from build123d import *

# Parameters (mm, degrees)
F0_R     = 38.1
F1_DEPTH = 6.35
F2_W     = 23.521014
F2_H     = 14.845229
F3_DEPTH = 5.842
F4_R     = 5.483658
F5_DEPTH = 27.94


with BuildPart() as f1:
    # F0 (on Top) → F1 (new body)
    with BuildSketch(Plane.XY):
        Circle(F0_R)
    extrude(amount=F1_DEPTH)

    # F2 (on face) → F3 (join)
    with BuildSketch(Plane.XY.offset(6.35)):
        with Locations((0.192795, 17.737156)):
            Rectangle(F2_W, F2_H)
    extrude(amount=F3_DEPTH)

    # F4 (on face) → F5 (cut)
    with BuildSketch(Plane.XY.offset(12.192)):
        with Locations((0, 17.833555)):
            Circle(F4_R)
    extrude(amount=-F5_DEPTH, mode=Mode.SUBTRACT)


solid = f1.part
Geometry: final body of the model. Coordinates: model frame, mm. A direction names the side the tool comes from. Round coordinates to 2 decimals unless told otherwise and drop trailing zeros. Loops run counter-clockwise (first coordinate to the right, second up) from the corner with the lowest first, then second, coordinate; pieces in that order, holes last. Notation, with made-up numbers: (41, 69.5) - (96, 69.5) arc R20 ccw to (96, 101.5) - close; hole circle Ø11 at (49.5, 6.25). An arc over 180 degrees is marked (long way). Write each question's results on one line, items separated by ' | '. Start each with the question number.
1) Access query for faces 1 (the face through (11.953, 18, 9)), 2 (the face through (-11.568, 18, 9)), 3 (the face through (0, 10.315, 9)), 4 (the face through (0, 25.16, 9)). Directions: +Z, -Z, +X, -X, +Y, -Y. A direction counts if a zero-diameter tool reaches every point of the face in a straight line with its end or side. Return the directions, or none.
2) Cut plane D-D on x = -10. Return loops of the section in (y, z).
3) Cut plane A-A on x = 0. Return loops of the section in (y, z).
4) Cut plane B-B on y = 0. Return loops of the section in (x, z), then the cut area to 3 significant figures.
5) Cut plane C-C on z = 1.75. Return loops of the section in (x, y), then the cut area to 3 significant figures.
6) Line query: probe 1 along Y at (x, z) = (0, 7.75); probe 2 along Z at (x, y) = (25, 17); probe 3 along Y at (x, z) = (0, 4). Output: solid intervals per line, ascending. Write a range as [from, to].
7) Mould query, pull axis X, two halves, no side actions, for faces 5 (the face through (-1.19, 12.48, 6.18)), 6 (the face through (-30.235, -23.183, 3.131)), 7 (the face through (-1, 1, 6.35)). Classes: released by +X, released by -X, zero draft, split by the parting line, or undercut.
8) First-contact query: P1, Ø12, axis at x = 16.5, y = -23, coming from the +Z side; P2, Ø4.5, axis at x = 3, z = 10.5, coming from the -Y side; P3, Ø1.5, axis at x = 4, z = 3.5, coming from the -Y side; P4, Ø6.5, axis at x = 0, y = 17.83, coming from the -Z side. Flat tips, straight axial feed; report the tip coordinate or a pass-through.
Verdict:
1) face 1: +Z, +X, +Y, -Y | face 2: +Z, -X, +Y, -Y | face 3: +Z, +X, -X, -Y | face 4: +Z, +X, -X, +Y
2) outline: (-36.76, 0) - (36.76, 0) - (36.76, 6.35) - (25.16, 6.35) - (25.16, 12.19) - (10.31, 12.19) - (10.31, 6.35) - (-36.76, 6.35) - close
3) outline: (-38.1, 0) - (12.35, 0) - (12.35, 12.19) - (10.31, 12.19) - (10.31, 6.35) - (-38.1, 6.35) - close; (23.32, 0) - (38.1, 0) - (38.1, 6.35) - (25.16, 6.35) - (25.16, 12.19) - (23.32, 12.19) - close
4) outline: (-38.1, 0) - (38.1, 0) - (38.1, 6.35) - (-38.1, 6.35) - close | area: 484 mm2
5) outline: circle Ø76.2 at (0, 0); hole circle Ø10.97 at (0, 17.83) | area: 4,470 mm2
6) probe 1: y = [10.31, 12.35], [23.32, 25.16] | probe 2: z = [0, 6.35] | probe 3: y = [-38.1, 12.35], [23.32, 38.1]
7) face 5: undercut | face 6: split by the parting line | face 7: zero draft
8) P1: stops at z = 6.35 | P2: stops at y = 10.31 | P3: stops at y = -37.96 | P4: passes through
